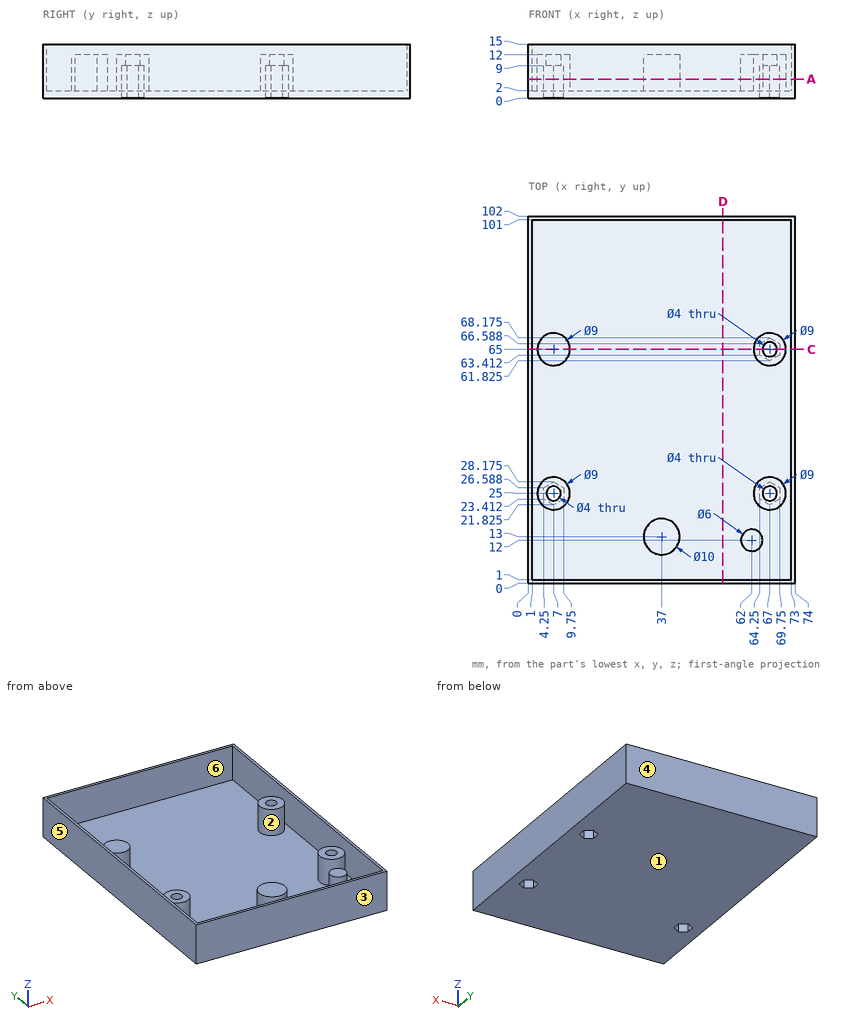
For this review, use the dimensioned drawing (mm, ordinates from the lowest corner) and the shaded views. A direction names the side the tool comes from. Round coordinates to 2 decimals unless told otherwise and drop trailing zeros. Write each loop counter-clockwise with the first axis right and the second up, starting at its lowest first coordinate (ties: lowest second). Pieces come first, ordered by that corner, then holes. Notation, with made-up numbers: (-29.5, 85) - (25.5, 85) arc R27 cw to (25.5, 101) - close; hole circle Ø8 at (5, 27). An arc over 180 degrees is marked (long way). Answer as a JSON object with one key per item and string values.
1. We need section C-C on y = 65. Give the boundary of the cut face in (x, z).
Response values:
{"outline": "(0, 0) - (64.25, 0) - (64.25, 9) - (65, 9) - (65, 12) - (62.5, 12) - (62.5, 2) - (11.5, 2) - (11.5, 12) - (2.5, 12) - (2.5, 2) - (1, 2) - (1, 15) - (0, 15) - close; (69, 9) - (69.75, 9) - (69.75, 0) - (74, 0) - (74, 15) - (73, 15) - (73, 2) - (71.5, 2) - (71.5, 12) - (69, 12) - close"}
2. Draft analysis for pull direction Y (two halves, no side actions). For the marked faces 3, 4, 5 and 6, state which applies: +Y half, -Y half, draft (parallel to the pull), parting line (faces both ways), or undercut.
Response values:
{"face 3": "-Y half", "face 4": "+Y half", "face 5": "draft", "face 6": "undercut"}
3. We need section A-A on z = 5.25. Count the separate pieces of the cut face and the enclosed holes in it.
Response values:
{"separate pieces": "7", "enclosed holes": "4"}
4. We need section D-D on x = 54. Give the boundary of the cut face in (y, z).
Response values:
{"outline": "(0, 0) - (102, 0) - (102, 15) - (101, 15) - (101, 2) - (1, 2) - (1, 15) - (0, 15) - close"}
5. To check wall thickness, follow line 1 along Y through (x, z) = (67, 9.8); line 2 along Y through (x, z) = (7, 9.7); line 3 along X through (y, z) = (66, 7.5). State the ranges of each line that lie inside material, in increasing order.
Response values:
{"line 1": "y = 0 to 1, 20.5 to 23, 27 to 29.5, 60.5 to 63, 67 to 69.5, 101 to 102", "line 2": "y = 0 to 1, 20.5 to 23, 27 to 29.5, 60.5 to 69.5, 101 to 102", "line 3": "x = 0 to 1, 2.61 to 11.39, 62.61 to 64.25, 69.75 to 71.39, 73 to 74"}
6. For pin 1 Ø4.5 at (x, y) = (67, 25) entering from -Z; pin 2 Ø2.5 at (x, y) = (67, 65) entering from -Z; pin 3 Ø10 at (x, y) = (8, 23) entering from +Z, all flat-tipped, find the tip position at first contact; note any pin that passes through.
Response values:
{"pin 1": "stops at z = 9", "pin 2": "passes through", "pin 3": "stops at z = 12"}
7. Tool access review of the marked faces 1 and 2: name each direction out of +Z, -Z, +X, -X, +Y, -Y from which nothing blocks a thin tool from reaching the whole face with its end or side.
Response values:
{"face 1": "-Z, +X, -X, +Y, -Y", "face 2": "+Z"}
